The model under review builds one solid part; all positions refer to its coordinate system, in mm. A direction names the side the tool comes from. Round coordinates to 2 decimals unless told otherwise and drop trailing zeros. Write each loop counter-clockwise with the first axis right and the second up, starting at its lowest first coordinate (ties: lowest second). Pieces come first, ordered by that corner, then holes. Notation, with made-up numbers: (40.5, 49.5) -> (96.5, 49.5) arc R20 ccw to (96.5, 64.5) -> close; hole circle Ø1 at (23.25, -12). An arc over 180 degrees is marked (long way). Answer as a JSON object with one key per item and string values. Group by question number.
1) To check wall thickness, follow probe 1 along X at (y, z) = (-14, 7.5); probe 2 along Y at (x, z) = (17, 3.5); probe 3 along Y at (x, z) = (-17, 7). State the ranges of each line that lie inside material, in increasing order. Write a range as [from, to].
2) Insertion check: pin 1 Ø1.3 at (x, z) = (-17.5, 6.5) entering from -Y; pin 2 Ø0.8 at (y, z) = (-17, 3.5) entering from +X; pin 3 Ø5 at (y, z) = (5.5, 5) entering from +X. Each pin has a flat end and moves straight along its axis. Give the tip position at first contact, or say it passes through.
3) Machinability: for faces 4 (the flat face through (5.753, 16.472, 5.134)), 5 (the flat face through (16.042, -7.725, 5.134)), 6 (the flat face through (0, -18, 5)), which of the approach directions +Z, -Z, +X, -X, +Y, -Y give a long, thin tool a straight path to every point of the face, cutting with its end or side? Answer none if there is none.
4) We need section A-A, the plane y = -1. Write out the cut boundary in (x, z) (1 decimal), then the cut area to 3 significant figures.
5) Mouldability with a two-part tool opening along X and no side actions: class faces 1 (the flat face through (-11.1, 13.92, 5.13)), 2 (the cylindrical face through (16.624, -9.304, 5.134)), 3 (the flat face through (-17.359, 3.962, 5.134)) as pulls with the +X half, pulls with the -X half, needs draft (parallel to the pull), parting line crosses it, or undercut.
from build123d import *

# Parameters (mm, degrees)
SKETCH1_R           = 19.05
BOSS_EXTRUDE1_DEPTH = 10.414
CUT_EXTRUDE1_DEPTH  = 10.414
CUT_EXTRUDE2_START  = -127
CUT_EXTRUDE2_DEPTH  = 127


with BuildPart() as part:
    # Sketch1 → Boss-Extrude1 (new body)
    with BuildSketch(Plane.XY):
        Circle(SKETCH1_R)
    extrude(amount=BOSS_EXTRUDE1_DEPTH)

    # Sketch2 → Cut-Extrude1 (cut)
    with BuildSketch(Plane.XY.offset(10.414)):
        Polygon((-7.332348419, 0), (-3.666174209, -6.35), (3.666174209, -6.35), (7.332348419, 0), (3.666174209, 6.35), (-3.666174209, 6.35), align=None)
    extrude(amount=-CUT_EXTRUDE1_DEPTH, mode=Mode.SUBTRACT)

    # Sketch3 → Cut-Extrude2 (cut)
    with BuildSketch(Plane.XY.offset(10.414).offset(CUT_EXTRUDE2_START)):
        with BuildLine():
            Line((0, 19.05), (0, 16.525205144))
            Line((0, 16.525205144), (-1.963187207, 16.262621871))
            Line((-1.963187207, 16.262621871), (-1.963187207, 18.9485724))
            ThreePointArc((-1.963187207, 18.9485724), (-0.982902788, 19.024626202), (0, 19.05))
        make_face()
        with BuildLine():
            Line((3.677204083, 16.11088375), (1.595179024, 15.811419173))
            Line((1.595179024, 15.811419173), (2.302488023, 18.910342379))
            ThreePointArc((2.302488023, 18.910342379), (3.275118227, 18.766355549), (4.239023792, 18.572376727))
            Line((4.239023792, 18.572376727), (3.677204083, 16.11088375))
        make_face()
        with BuildLine():
            Line((7.170017798, 14.888695371), (5.073556317, 15.060033157))
            Line((5.073556317, 15.060033157), (6.452706889, 17.923868829))
            ThreePointArc((6.452706889, 17.923868829), (7.368911139, 17.567061468), (8.26548523, 17.163456934))
            Line((8.26548523, 17.163456934), (7.170017798, 14.888695371))
        make_face()
        with BuildLine():
            Line((10.303296881, 12.919925636), (8.297524311, 13.553474193))
            Line((8.297524311, 13.553474193), (10.279360087, 16.038617653))
            ThreePointArc((10.279360087, 16.038617653), (11.093196077, 15.486881571), (11.877480725, 14.893889741))
            Line((11.877480725, 14.893889741), (10.303296881, 12.919925636))
        make_face()
        with BuildLine():
            Line((12.919925636, 10.303296881), (11.105419788, 11.367287439))
            Line((11.105419788, 11.367287439), (13.590563248, 13.349123215))
            ThreePointArc((13.590563248, 13.349123215), (14.261221842, 12.630124765), (14.893889741, 11.877480725))
            Line((14.893889741, 11.877480725), (12.919925636, 10.303296881))
        make_face()
        with BuildLine():
            Line((14.888695371, 7.170017798), (13.356443146, 8.611097427))
            Line((13.356443146, 8.611097427), (16.220278818, 9.990247999))
            ThreePointArc((16.220278818, 9.990247999), (16.714130394, 9.140040764), (17.163456934, 8.26548523))
            Line((17.163456934, 8.26548523), (14.888695371, 7.170017798))
        make_face()
        with BuildLine():
            Line((16.11088375, 3.677204083), (14.937718672, 5.423111033))
            Line((14.937718672, 5.423111033), (18.036641878, 6.130420032))
            ThreePointArc((18.036641878, 6.130420032), (18.328922656, 5.191636954), (18.572376727, 4.239023792))
            Line((18.572376727, 4.239023792), (16.11088375, 3.677204083))
        make_face()
        with BuildLine():
            Line((16.525205144, 0), (15.76995461, 1.963187207))
            Line((15.76995461, 1.963187207), (18.9485724, 1.963187207))
            ThreePointArc((18.9485724, 1.963187207), (19.024626202, 0.982902788), (19.05, 0))
            Line((19.05, 0), (16.525205144, 0))
        make_face()
        with BuildLine():
            Line((16.11088375, -3.677204083), (15.811419173, -1.595179024))
            Line((15.811419173, -1.595179024), (18.910342379, -2.302488023))
            ThreePointArc((18.910342379, -2.302488023), (18.766355549, -3.275118227), (18.572376727, -4.239023792))
            Line((18.572376727, -4.239023792), (16.11088375, -3.677204083))
        make_face()
        with BuildLine():
            Line((14.888695371, -7.170017798), (15.060033157, -5.073556317))
            Line((15.060033157, -5.073556317), (17.923868829, -6.452706889))
            ThreePointArc((17.923868829, -6.452706889), (17.567061468, -7.368911139), (17.163456934, -8.26548523))
            Line((17.163456934, -8.26548523), (14.888695371, -7.170017798))
        make_face()
        with BuildLine():
            Line((12.919925636, -10.303296881), (13.553474193, -8.297524311))
            Line((13.553474193, -8.297524311), (16.038617653, -10.279360087))
            ThreePointArc((16.038617653, -10.279360087), (15.486881571, -11.093196077), (14.893889741, -11.877480725))
            Line((14.893889741, -11.877480725), (12.919925636, -10.303296881))
        make_face()
        with BuildLine():
            Line((10.303296881, -12.919925636), (11.367287439, -11.105419788))
            Line((11.367287439, -11.105419788), (13.349123215, -13.590563248))
            ThreePointArc((13.349123215, -13.590563248), (12.630124765, -14.261221842), (11.877480725, -14.893889741))
            Line((11.877480725, -14.893889741), (10.303296881, -12.919925636))
        make_face()
        with BuildLine():
            Line((7.170017798, -14.888695371), (8.611097427, -13.356443146))
            Line((8.611097427, -13.356443146), (9.990247999, -16.220278818))
            ThreePointArc((9.990247999, -16.220278818), (9.140040764, -16.714130394), (8.26548523, -17.163456934))
            Line((8.26548523, -17.163456934), (7.170017798, -14.888695371))
        make_face()
        with BuildLine():
            Line((3.677204083, -16.11088375), (5.423111033, -14.937718672))
            Line((5.423111033, -14.937718672), (6.130420032, -18.036641878))
            ThreePointArc((6.130420032, -18.036641878), (5.191636954, -18.328922656), (4.239023792, -18.572376727))
            Line((4.239023792, -18.572376727), (3.677204083, -16.11088375))
        make_face()
        with BuildLine():
            Line((0, -16.525205144), (1.963187207, -15.76995461))
            Line((1.963187207, -15.76995461), (1.963187207, -18.9485724))
            ThreePointArc((1.963187207, -18.9485724), (0.982902788, -19.024626202), (0, -19.05))
            Line((0, -19.05), (0, -16.525205144))
        make_face()
        with BuildLine():
            Line((-3.677204083, -16.11088375), (-1.595179024, -15.811419173))
            Line((-1.595179024, -15.811419173), (-2.302488023, -18.910342379))
            ThreePointArc((-2.302488023, -18.910342379), (-3.275118227, -18.766355549), (-4.239023792, -18.572376727))
            Line((-4.239023792, -18.572376727), (-3.677204083, -16.11088375))
        make_face()
        with BuildLine():
            Line((-7.170017798, -14.888695371), (-5.073556317, -15.060033157))
            Line((-5.073556317, -15.060033157), (-6.452706889, -17.923868829))
            ThreePointArc((-6.452706889, -17.923868829), (-7.368911139, -17.567061468), (-8.26548523, -17.163456934))
            Line((-8.26548523, -17.163456934), (-7.170017798, -14.888695371))
        make_face()
        with BuildLine():
            Line((-10.303296881, -12.919925636), (-8.297524311, -13.553474193))
            Line((-8.297524311, -13.553474193), (-10.279360087, -16.038617653))
            ThreePointArc((-10.279360087, -16.038617653), (-11.093196077, -15.486881571), (-11.877480725, -14.893889741))
            Line((-11.877480725, -14.893889741), (-10.303296881, -12.919925636))
        make_face()
        with BuildLine():
            Line((-12.919925636, -10.303296881), (-11.105419788, -11.367287439))
            Line((-11.105419788, -11.367287439), (-13.590563248, -13.349123215))
            ThreePointArc((-13.590563248, -13.349123215), (-14.261221842, -12.630124765), (-14.893889741, -11.877480725))
            Line((-14.893889741, -11.877480725), (-12.919925636, -10.303296881))
        make_face()
        with BuildLine():
            Line((-14.888695371, -7.170017798), (-13.356443146, -8.611097427))
            Line((-13.356443146, -8.611097427), (-16.220278818, -9.990247999))
            ThreePointArc((-16.220278818, -9.990247999), (-16.714130394, -9.140040764), (-17.163456934, -8.26548523))
            Line((-17.163456934, -8.26548523), (-14.888695371, -7.170017798))
        make_face()
        with BuildLine():
            Line((-16.11088375, -3.677204083), (-14.937718672, -5.423111033))
            Line((-14.937718672, -5.423111033), (-18.036641878, -6.130420032))
            ThreePointArc((-18.036641878, -6.130420032), (-18.328922656, -5.191636954), (-18.572376727, -4.239023792))
            Line((-18.572376727, -4.239023792), (-16.11088375, -3.677204083))
        make_face()
        with BuildLine():
            Line((-16.525205144, 0), (-15.76995461, -1.963187207))
            Line((-15.76995461, -1.963187207), (-18.9485724, -1.963187207))
            ThreePointArc((-18.9485724, -1.963187207), (-19.024626202, -0.982902788), (-19.05, 0))
            Line((-19.05, 0), (-16.525205144, 0))
        make_face()
        with BuildLine():
            Line((-16.11088375, 3.677204083), (-15.811419173, 1.595179024))
            Line((-15.811419173, 1.595179024), (-18.910342379, 2.302488023))
            ThreePointArc((-18.910342379, 2.302488023), (-18.766355549, 3.275118227), (-18.572376727, 4.239023792))
            Line((-18.572376727, 4.239023792), (-16.11088375, 3.677204083))
        make_face()
        with BuildLine():
            Line((-14.888695371, 7.170017798), (-15.060033157, 5.073556317))
            Line((-15.060033157, 5.073556317), (-17.923868829, 6.452706889))
            ThreePointArc((-17.923868829, 6.452706889), (-17.567061468, 7.368911139), (-17.163456934, 8.26548523))
            Line((-17.163456934, 8.26548523), (-14.888695371, 7.170017798))
        make_face()
        with BuildLine():
            Line((-12.919925636, 10.303296881), (-13.553474193, 8.297524311))
            Line((-13.553474193, 8.297524311), (-16.038617653, 10.279360087))
            ThreePointArc((-16.038617653, 10.279360087), (-15.486881571, 11.093196077), (-14.893889741, 11.877480725))
            Line((-14.893889741, 11.877480725), (-12.919925636, 10.303296881))
        make_face()
        with BuildLine():
            Line((-10.303296881, 12.919925636), (-11.367287439, 11.105419788))
            Line((-11.367287439, 11.105419788), (-13.349123215, 13.590563248))
            ThreePointArc((-13.349123215, 13.590563248), (-12.630124765, 14.261221842), (-11.877480725, 14.893889741))
            Line((-11.877480725, 14.893889741), (-10.303296881, 12.919925636))
        make_face()
        with BuildLine():
            Line((-7.170017798, 14.888695371), (-8.611097427, 13.356443146))
            Line((-8.611097427, 13.356443146), (-9.990247999, 16.220278818))
            ThreePointArc((-9.990247999, 16.220278818), (-9.140040764, 16.714130394), (-8.26548523, 17.163456934))
            Line((-8.26548523, 17.163456934), (-7.170017798, 14.888695371))
        make_face()
        with BuildLine():
            Line((-3.677204083, 16.11088375), (-5.423111033, 14.937718672))
            Line((-5.423111033, 14.937718672), (-6.130420032, 18.036641878))
            ThreePointArc((-6.130420032, 18.036641878), (-5.191636954, 18.328922656), (-4.239023792, 18.572376727))
            Line((-4.239023792, 18.572376727), (-3.677204083, 16.11088375))
        make_face()
    extrude(amount=CUT_EXTRUDE2_DEPTH, mode=Mode.SUBTRACT)


solid = part.part
Here are the results:
{
 "1": {"probe 1": "x = [-12.92, -11.16], [-8.65, 8.01], [8.92, 11.16]", "probe 2": "y = [-8.6, -8.19], [-6.01, -3.88], [-1.87, 0], [1.96, 3.88], [5.89, 8.19]", "probe 3": "y = [-8.19, -5.89], [-3.88, -1.96], [0, 1.87], [3.88, 6.01], [8.19, 8.6]"},
 "2": {"pin 1": "stops at y = -8.27", "pin 2": "stops at x = 8.27", "pin 3": "stops at x = 18.81"},
 "3": {"face 4": "+Z, -Z", "face 5": "+Z, -Z, +X", "face 6": "+Z, -Z, -Y"},
 "4": {"outline": "(-16.1, 0) -> (-6.8, 0) -> (-6.8, 10.4) -> (-16.1, 10.4) -> close; (6.8, 0) -> (19, 0) -> (19, 10.4) -> (6.8, 10.4) -> close", "area": "226 mm^2"},
 "5": {"face 1": "undercut", "face 2": "pulls with the +X half", "face 3": "pulls with the -X half"}
}
